Read the model definition and answer for the solid it produces. Units are mm, in the model's axes. Face numbers are marked on the shaded views. A direction names the side the tool comes from. Round coordinates to 2 decimals unless told otherwise and drop trailing zeros. Write each loop counter-clockwise with the first axis right and the second up, starting at its lowest first coordinate (ties: lowest second). Pieces come first, ordered by that corner, then holes. Notation, with made-up numbers: (-19, -33) -> (4, -33) arc R18 ccw to (4, -23) -> close; hole circle Ø3 at (87.25, 32). An arc over 180 degrees is marked (long way). Return JSON: item names as keys, results as strings.
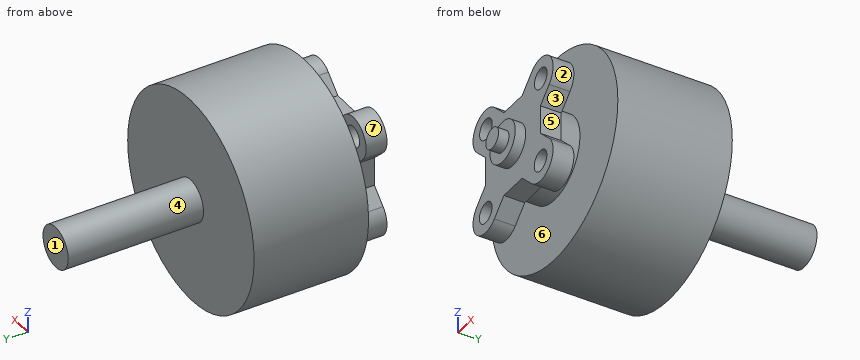
from build123d import *

# Parameters (mm, degrees)
SKETCH2_R           = 10
BOSS_EXTRUDE2_DEPTH = 30
CUT_EXTRUDE5_START  = -13
SKETCH8_R           = 10
SKETCH8_R_2         = 4
CUT_EXTRUDE5_DEPTH  = 13
CUT_EXTRUDE6_START  = -13
SKETCH9_R           = 4
SKETCH9_R_2         = 2
CUT_EXTRUDE6_DEPTH  = 13
SKETCH10_R          = 10
SKETCH10_R_2        = 1
CUT_EXTRUDE7_DEPTH  = 1
SKETCH11_R          = 10
SKETCH11_R_2        = 2
CUT_EXTRUDE8_DEPTH  = 2
SKETCH12_R          = 10
CUT_EXTRUDE9_DEPTH  = 4
SKETCH13_R          = 10
SKETCH13_R_2        = 4
CUT_EXTRUDE10_DEPTH = 2
SKETCH14_R          = 1
CUT_EXTRUDE11_DEPTH = 2


with BuildPart() as part:
    # Sketch2 → Boss-Extrude2 (new body)
    with BuildSketch(Plane(origin=(0, 0, 0), x_dir=(1, 0, 0), z_dir=(0, 1, 0))):
        with Locations(Location((0, 0, 0), (0, 0, 270))):
            Circle(SKETCH2_R)
    extrude(amount=BOSS_EXTRUDE2_DEPTH)

    # Sketch8 → Cut-Extrude5 (cut)
    with BuildSketch(Plane(origin=(0, 30, 0), x_dir=(1, 0, 0), z_dir=(0, 1, 0)).offset(CUT_EXTRUDE5_START)):
        with Locations(Location((0, 0, 0), (0, 0, 270))):
            Circle(SKETCH8_R)
        with Locations(Location((0, 0, 0), (0, 0, 270))):
            Circle(SKETCH8_R_2, mode=Mode.SUBTRACT)
    extrude(amount=CUT_EXTRUDE5_DEPTH, mode=Mode.SUBTRACT)

    # Sketch9 → Cut-Extrude6 (cut)
    with BuildSketch(Plane(origin=(0, 30, 0), x_dir=(1, 0, 0), z_dir=(0, 1, 0)).offset(CUT_EXTRUDE6_START)):
        Circle(SKETCH9_R)
        with Locations(Location((0, 0, 0), (0, 0, 270))):
            Circle(SKETCH9_R_2, mode=Mode.SUBTRACT)
    extrude(amount=CUT_EXTRUDE6_DEPTH, mode=Mode.SUBTRACT)

    # Sketch10 → Cut-Extrude7 (cut)
    with BuildSketch(Plane.XZ):
        with Locations(Location((0, 0, 0), (0, 0, 270))):
            Circle(SKETCH10_R)
        with Locations(Location((0, 0, 0), (0, 0, 270))):
            Circle(SKETCH10_R_2, mode=Mode.SUBTRACT)
    extrude(amount=-CUT_EXTRUDE7_DEPTH, mode=Mode.SUBTRACT)

    # Sketch11 → Cut-Extrude8 (cut)
    with BuildSketch(Plane(origin=(0, 0, 0), x_dir=(-1, 0, 0), z_dir=(0, -1, 0))):
        with Locations(Location((0, 0, 0), (0, 0, 90))):
            Circle(SKETCH11_R)
        with Locations(Location((0, 0, 0), (0, 0, 270))):
            Circle(SKETCH11_R_2, mode=Mode.SUBTRACT)
    extrude(amount=-CUT_EXTRUDE8_DEPTH, mode=Mode.SUBTRACT)

    # Sketch12 → Cut-Extrude9 (cut)
    with BuildSketch(Plane(origin=(0, 0, 0), x_dir=(-1, 0, 0), z_dir=(0, -1, 0))):
        with Locations(Location((0, 0, 0), (0, 0, 90))):
            Circle(SKETCH12_R)
        with BuildLine():
            Line((1.442076294, -4.148689545), (-1.442076294, -4.148689545))
            Line((-1.442076294, -4.148689545), (-2.95165941, -5.593541519))
            ThreePointArc((-2.95165941, -5.593541519), (-5.779407899, -5.53158606), (-5.717452439, -2.70383757))
            Line((-5.717452439, -2.70383757), (-4.334555924, -1.380239856))
            Line((-4.334555924, -1.380239856), (-4.334555924, 1.380239856))
            Line((-4.334555924, 1.380239856), (-5.717452439, 2.70383757))
            ThreePointArc((-5.717452439, 2.70383757), (-5.779407899, 5.53158606), (-2.95165941, 5.593541519))
            Line((-2.95165941, 5.593541519), (-1.442076294, 4.148689545))
            Line((-1.442076294, 4.148689545), (1.442076294, 4.148689545))
            Line((1.442076294, 4.148689545), (2.95165941, 5.593541519))
            ThreePointArc((2.95165941, 5.593541519), (5.779407899, 5.53158606), (5.717452439, 2.70383757))
            Line((5.717452439, 2.70383757), (4.334555924, 1.380239856))
            Line((4.334555924, 1.380239856), (4.334555924, -1.380239856))
            Line((4.334555924, -1.380239856), (5.717452439, -2.70383757))
            ThreePointArc((5.717452439, -2.70383757), (5.779407899, -5.53158606), (2.95165941, -5.593541519))
            Line((2.95165941, -5.593541519), (1.442076294, -4.148689545))
        make_face(mode=Mode.SUBTRACT)
    extrude(amount=-CUT_EXTRUDE9_DEPTH, mode=Mode.SUBTRACT)

    # Sketch13 → Cut-Extrude10 (cut)
    with BuildSketch(Plane.XZ.offset(-4)):
        with Locations(Location((0, 0, 0), (0, 0, 270))):
            Circle(SKETCH13_R)
        with Locations(Location((0, 0, 0), (0, 0, 270))):
            Circle(SKETCH13_R_2, mode=Mode.SUBTRACT)
    extrude(amount=-CUT_EXTRUDE10_DEPTH, mode=Mode.SUBTRACT)

    # Sketch14 → Cut-Extrude11 (cut)
    with BuildSketch(Plane.XZ.offset(-2)):
        with Locations(Location((-4.287533824, 4.199553123, 0), (0, 0, 270))):
            Circle(SKETCH14_R)
        with Locations(Location((4.390527215, 4.092485492, 0), (0, 0, 270))):
            Circle(SKETCH14_R)
        with Locations(Location((4.354750155, -4.127894387, 0), (0, 0, 270))):
            Circle(SKETCH14_R)
        with Locations(Location((-4.322800784, -4.16107677, 0), (0, 0, 270))):
            Circle(SKETCH14_R)
    extrude(amount=-CUT_EXTRUDE11_DEPTH, mode=Mode.SUBTRACT)


solid = part.part
Item 1: Section B-B (x = 4.75) is taken. Give the vertices of the cut face in (y, z), then the cut area to 3 significant figures.
Worked answers:
{"outline": "(2, -6.11) -> (4, -6.11) -> (4, -5.05) -> (2, -5.05) -> close; (2, -3.21) -> (4, -3.21) -> (4, -1.78) -> (2, -1.78) -> close; (2, 1.78) -> (4, 1.78) -> (4, 3.16) -> (2, 3.16) -> close; (2, 5.03) -> (4, 5.03) -> (4, 6.11) -> (2, 6.11) -> close; (6, -8.8) -> (17, -8.8) -> (17, 8.8) -> (6, 8.8) -> close", "area": "203 mm2"}
Item 2: A tool of negligible diameter and unlimited length cuts with its end or side. For the marked faces 5, 6 and 7, from which of +Z, -Z, +X, -X, +Y, -Y can it reach the whole face along a straight path? Write none if from no direction.
Worked answers:
{"face 5": "+X, -Y", "face 6": "none", "face 7": "-Y"}
Item 3: Straight lines are drawn through the part: L1, parallel to Y at x = -5, z = 3; L2, parallel to Y at x = -7.5, z = -0.5; L3, parallel to X at y = 21, z = 0. For each, find the intervals that lie inside material, in ascending order. Write a range as [from, to].
Worked answers:
{"L1": "y = [2, 4], [6, 17]", "L2": "y = [6, 17]", "L3": "x = [-2, 2]"}
Item 4: Section A-A (x = 0) is taken. Give the vertices of the cut face in (y, z), then the cut area to 3 significant figures.
Worked answers:
{"outline": "(0, -1) -> (1, -1) -> (1, -2) -> (2, -2) -> (2, -4.15) -> (4, -4.15) -> (4, -4) -> (6, -4) -> (6, -10) -> (17, -10) -> (17, -2) -> (30, -2) -> (30, 2) -> (17, 2) -> (17, 10) -> (6, 10) -> (6, 4) -> (4, 4) -> (4, 4.15) -> (2, 4.15) -> (2, 2) -> (1, 2) -> (1, 1) -> (0, 1) -> close", "area": "311 mm2"}
Item 5: Section C-C (z = 0) is taken. Give the vertices of the cut face in (x, y).
Worked answers:
{"outline": "(-10, 6) -> (-4, 6) -> (-4, 4) -> (-4.33, 4) -> (-4.33, 2) -> (-2, 2) -> (-2, 1) -> (-1, 1) -> (-1, 0) -> (1, 0) -> (1, 1) -> (2, 1) -> (2, 2) -> (4.33, 2) -> (4.33, 4) -> (4, 4) -> (4, 6) -> (10, 6) -> (10, 17) -> (2, 17) -> (2, 30) -> (-2, 30) -> (-2, 17) -> (-10, 17) -> close"}
Item 6: For a pull along Z with two mould halves and no side action, classify the marked faces 1, 2, 3 and 4 as released by +Z, released by -Z, zero draft, split by the parting line, or undercut.
Worked answers:
{"face 1": "zero draft", "face 2": "undercut", "face 3": "undercut", "face 4": "split by the parting line"}
Item 7: Flat-ended cylindrical pins translate along their axes: pin 1 (1.6 mm diameter, centred on x = -4.29, z = 4.2, fed in from -Y); pin 2 (2.5 mm diameter, centred on x = 4.35, z = -4.13, fed in from +Y); pin 3 (2 mm diameter, centred on y = 3, z = -0.5, fed in from -X); pin 4 (6 mm diameter, centred on y = 25, z = 6, fed in from +X). Find the tip coordinate at first contact, or state that the pin passes through.
Worked answers:
{"pin 1": "stops at y = 6", "pin 2": "stops at y = 17", "pin 3": "stops at x = -4.46", "pin 4": "passes through"}
Item 8: Section D-D (y = 21) is taken. Give the vertices of the cut face in (x, z).
Worked answers:
{"outline": "circle Ø4 at (0, 0)"}
